Build history of the part. All positions in model axes, mm. A direction names the side the tool comes from. Round coordinates to 2 decimals unless told otherwise and drop trailing zeros. Order: outer loops, then holes, each group sorted by start corner. A loop starts at its lowest first (then second) coordinate and runs counter-clockwise, first axis right, second up. Notation, with made-up numbers: M -23.5,40.5 L -15.5,40.5 A29 ccw -15.5,67.5 Z; hole C -35,75.5 d3. An arc over 180 degrees is marked long. Use CSV: the item, a comma, the result in double quotes.
Autodesk Inventor part; units mm, degrees
ref_plane "YZ Plane" through (0, 0, 0) normal (1, 0, 0) x (0, 1, 0)
ref_plane "XZ Plane" through (0, 0, 0) normal (0, 1, 0) x (-1, 0, 0)
ref_plane "XY Plane" through (0, 0, 0) normal (0, 0, 1) x (1, 0, 0)
sketch "Sketch1" plane through (0, 0, 0) normal (0, 0, 1) x (1, 0, 0)
  line L0 (0, 0) -> (25.4, 0)
  line L1 (25.4, 0) -> (25.4, 25.4)
  line L2 (25.4, 25.4) -> (0, 25.4)
  line L3 (0, 25.4) -> (0, 0)
  line L4 (3.175, 22.225) -> (22.225, 22.225)
  line L5 (22.225, 22.225) -> (22.225, 3.175)
  line L6 (22.225, 3.175) -> (3.175, 3.175)
  line L7 (3.175, 3.175) -> (3.175, 22.225)
  dimension "d0" = 25.4
  dimension "d1" = 25.4
  dimension "d2" = 3.175
extrude "Extrusion1" add sketch "Sketch1" along normal blind 76.2
sketch "Sketch2" plane through (25.4, 0, 0) normal (1, 0, 0) x (0, 0, -1)
  line L0 (0, 0) -> (0, 25.4)
  line L1 (-76.2, 0) -> (-76.2, 25.4)
  line L2 (0, 25.4) -> (-76.2, 25.4)
  point P0 (-63.5, 12.7)
  point P1 (-12.7, 12.7)
  dimension "d5" = 12.7
  dimension "d6" = 12.7
  dimension "d7" = 12.7
  dimension "d8" = 12.7
hole "Hole1" at (25.4, 12.7, 63.5) at (25.4, 12.7, 12.7) direction (-1, 0, 0) diameter 5.1594 end through all
sketch "Sketch3" plane through (0, 25.4, 0) normal (0, 1, 0) x (1, 0, 0)
  line L0 (25.4, -76.2) -> (0, -76.2)
  line L1 (25.4, 0) -> (25.4, -76.2)
  point P0 (0, 0)
  point P1 (14.2875, -30.1498)
  dimension "d16" = 46.0502
  dimension "d17" = 11.1125
hole "Hole2" at (14.2875, 25.4, 30.1498) direction (0, -1, 0) diameter 6.7469 end through all
properties part number "1512898-16-A-0901"
(1) Wall check: line 1 (Z direction, x = 1.45, y = 12.7); line 2 (Y direction, x = 14.5, z = 45) (3 decimals); line 3 (Y direction, x = 1.7, z = 12.7). Give the ranges that are in metal, low to high. Write a range as from..to.
Answer block:
line 1,"z = 0..10.12, 15.28..60.92, 66.08..76.2"
line 2,"y = 0..3.175, 22.225..25.4"
line 3,"y = 0..10.12, 15.28..25.4"
(2) Two-plate mould, pull along Y, no slides. Class faces 3 (the face through (13, 22.225, 38)), 4 (the face through (13, 25.4, 38)), 5 (the face through (24, 13, 76.2)): released by +Y, released by -Y, zero draft, split by the parting line, or undercut.
Answer block:
face 3,"undercut"
face 4,"released by +Y"
face 5,"zero draft"
(3) Cut at D-D, the plane z = 45.5. Give the cut face in (x, y) (3 decimals), and give its area (3 significant figures).
Answer block:
outline,"M 0,0 L 25.4,0 L 25.4,25.4 L 0,25.4 Z; hole M 3.175,3.175 L 22.225,3.175 L 22.225,22.225 L 3.175,22.225 Z"
area,"282 mm²"
(4) Cut at A-A, the plane z = 63.5. Give the cut face in (x, y) (3 decimals), and give its area (3 significant figures).
Answer block:
outline,"M 0,0 L 25.4,0 L 25.4,10.12 L 22.225,10.12 L 22.225,3.175 L 3.175,3.175 L 3.175,10.12 L 0,10.12 Z; M 0,15.28 L 3.175,15.28 L 3.175,22.225 L 22.225,22.225 L 22.225,15.28 L 25.4,15.28 L 25.4,25.4 L 0,25.4 Z"
area,"249 mm²"
(5) Drop a flat-ended pin along its axis: pin 1 (6.5 mm diameter, centred on y = 12.7, z = 12.7, fed in from +X). Give the stop position or say it passes through.
Answer block:
pin 1,"stops at x = 25.4"
(6) Cut at C-C, the plane x = 20.25. Give the cut face in (y, z) (3 decimals).
Answer block:
outline,"M 0,0 L 3.175,0 L 3.175,76.2 L 0,76.2 Z; M 22.225,0 L 25.4,0 L 25.4,76.2 L 22.225,76.2 Z"
(7) Cut at B-B, the plane y = 12.7. Give the cut face in (x, z) (3 decimals).
Answer block:
outline,"M 0,0 L 3.175,0 L 3.175,10.12 L 0,10.12 Z; M 0,15.28 L 3.175,15.28 L 3.175,60.92 L 0,60.92 Z; M 0,66.08 L 3.175,66.08 L 3.175,76.2 L 0,76.2 Z; M 22.225,0 L 25.4,0 L 25.4,10.12 L 22.225,10.12 Z; M 22.225,15.28 L 25.4,15.28 L 25.4,60.92 L 22.225,60.92 Z; M 22.225,66.08 L 25.4,66.08 L 25.4,76.2 L 22.225,76.2 Z"
(8) Tool access for faces 1 (the face through (3.175, 13, 38)), 2 (the face through (17.28, 1.57, 31.71)): list every direction of +Z, -Z, +X, -X, +Y, -Y with a clear straight run to the whole face (end or side of a thin tool).
Answer block:
face 1,"+Z, -Z"
face 2,"+Y, -Y"
